The figure shows three views and two pictorial views of one solid part (mm, origin at its lowest corner). Answer the questions. Give positions to 0.01 mm unless a question says otherwise; leave off trailing zeros. Loops run counter-clockwise (first coordinate to the right, second up) from the corner with the lowest first, then second, coordinate; pieces in that order, holes last. Notation, with made-up numbers: (58.25, 53) - (117.25, 53) arc R25 ccw to (117.25, 68) - close; hole circle Ø7 at (-1, -5.5). An arc over 180 degrees is marked (long way). Use CSV: the item, a comma, the result in double quotes.
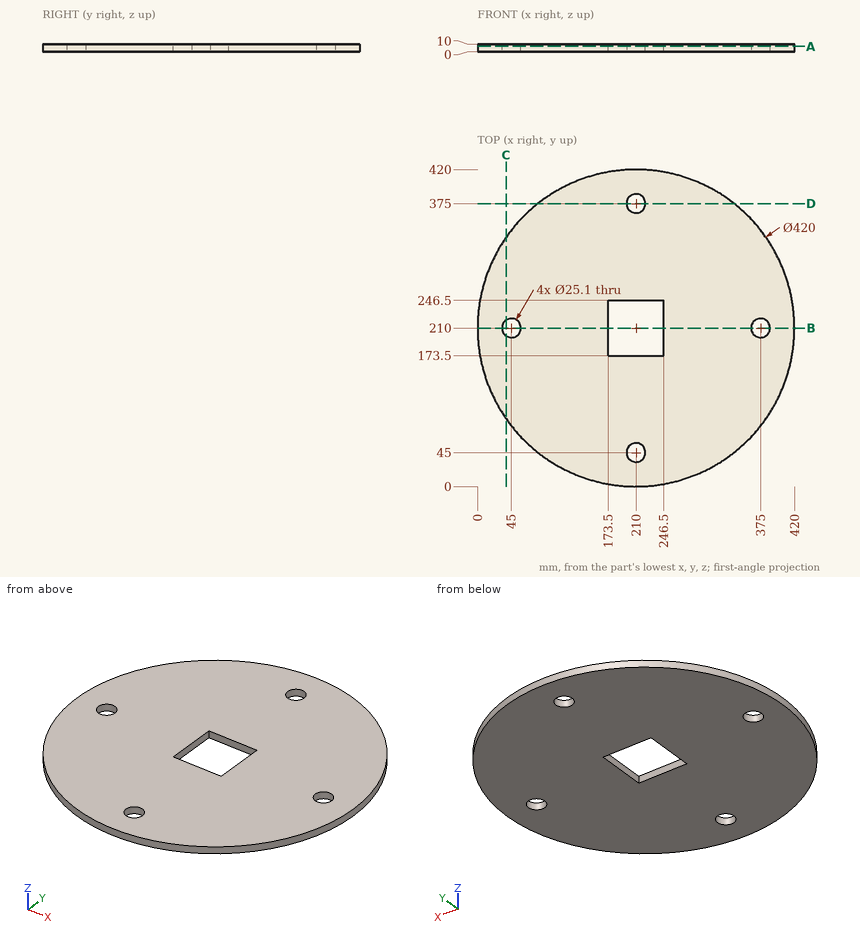
Item 1: A cutting plane is placed at B-B on y = 210. Determine the outline of the cut face in (x, z).
Determined:
outline,"(0, 0) - (32.45, 0) - (32.45, 10) - (0, 10) - close; (57.55, 0) - (173.5, 0) - (173.5, 10) - (57.55, 10) - close; (246.5, 0) - (362.45, 0) - (362.45, 10) - (246.5, 10) - close; (387.55, 0) - (420, 0) - (420, 10) - (387.55, 10) - close"
Item 2: A cutting plane is placed at A-A on z = 7. Determine the outline of the cut face in (x, y).
Determined:
outline,"circle Ø420 at (210, 210); hole circle Ø25.1 at (45, 210); hole (173.5, 173.5) - (246.5, 173.5) - (246.5, 246.5) - (173.5, 246.5) - close; hole circle Ø25.1 at (210, 45); hole circle Ø25.1 at (210, 375); hole circle Ø25.1 at (375, 210)"
Item 3: A cutting plane is placed at C-C on x = 38. Determine the outline of the cut face in (y, z), and give its area (3 significant figures).
Determined:
outline,"(89.52, 0) - (199.58, 0) - (199.58, 10) - (89.52, 10) - close; (220.42, 0) - (330.48, 0) - (330.48, 10) - (220.42, 10) - close"
area,"2,200 mm²"
Item 4: Find the intervals of material crossed by line 1 (Y direction, x = 210, z = 2.5); line 2 (Y direction, x = 375, z = 4); line 3 (Y direction, x = 178, z = 9), in increasing order.
Determined:
line 1,"y = 0 to 32.45, 57.55 to 173.5, 246.5 to 362.45, 387.55 to 420"
line 2,"y = 80.1 to 197.45, 222.55 to 339.9"
line 3,"y = 2.45 to 173.5, 246.5 to 417.55"
Item 5: A cutting plane is placed at D-D on y = 375. Determine the outline of the cut face in (x, z), and give its area (3 significant figures).
Determined:
outline,"(80.1, 0) - (197.45, 0) - (197.45, 10) - (80.1, 10) - close; (222.55, 0) - (339.9, 0) - (339.9, 10) - (222.55, 10) - close"
area,"2,350 mm²"
Item 6: Given P1, Ø1.5, axis at y = 327.5, z = 2, coming from the -X side; P2, Ø1.5, axis at x = 267.5, z = 3.5, coming from the -Y side; P3, Ø1, axis at y = 193, z = 5, coming from the +X side, each flat-ended and moving along its own axis, determine where each tip first touches the part or whether it passes through.
Determined:
P1,"stops at x = 35.45"
P2,"stops at y = 7.81"
P3,"stops at x = 419.35"
